from build123d import *

# Parameters (mm, degrees)
SKETCH1_W           = 160
SKETCH1_H           = 350
BOSS_EXTRUDE1_DEPTH = 3
SKETCH2_R           = 5
BOSS_EXTRUDE2_DEPTH = 20
SKETCH3_R           = 5
BOSS_EXTRUDE3_DEPTH = 20


with BuildPart() as part:
    # Sketch1 → Boss-Extrude1 (new body)
    with BuildSketch(Plane.XY):
        Rectangle(SKETCH1_W, SKETCH1_H)
    extrude(amount=BOSS_EXTRUDE1_DEPTH)

    # Sketch2 → Boss-Extrude2 (add)
    with BuildSketch(Plane.XY.offset(3)):
        with Locations((70, 150)):
            Circle(SKETCH2_R)
    boss_extrude2 = extrude(amount=BOSS_EXTRUDE2_DEPTH)

    # Mirror1: Boss-Extrude2 across plane
    add(boss_extrude2.mirror(Plane.ZX))

    # Sketch3 → Boss-Extrude3 (add)
    with BuildSketch(Plane.XY.offset(3)):
        with Locations((-60, 0)):
            Circle(SKETCH3_R)
    extrude(amount=BOSS_EXTRUDE3_DEPTH)


solid = part.part
Work out the finished part from the listing and answer in its coordinate system (mm). Round coordinates to 2 decimals unless told otherwise and drop trailing zeros. Write each loop counter-clockwise with the first axis right and the second up, starting at its lowest first coordinate (ties: lowest second). Pieces come first, ordered by that corner, then holes. Notation, with made-up numbers: (37.25, 40) -> (88.25, 40) arc R24 ccw to (88.25, 76) -> close; hole circle Ø7 at (12.25, 32.5). An arc over 180 degrees is marked (long way). Write each question's results on one line, items separated by ' | '.
Item 1: A cutting plane is placed at C-C, the plane x = 70. Determine the outline of the cut face in (y, z).
Result set:
outline: (-175, 0) -> (175, 0) -> (175, 3) -> (155, 3) -> (155, 23) -> (145, 23) -> (145, 3) -> (-145, 3) -> (-145, 23) -> (-155, 23) -> (-155, 3) -> (-175, 3) -> close
Item 2: A cutting plane is placed at B-B, the plane y = 150. Determine the outline of the cut face in (x, z), plus the area to 3 significant figures.
Result set:
outline: (-80, 0) -> (80, 0) -> (80, 3) -> (75, 3) -> (75, 23) -> (65, 23) -> (65, 3) -> (-80, 3) -> close | area: 680 mm^2
Item 3: A cutting plane is placed at D-D, the plane x = -60. Determine the outline of the cut face in (y, z), plus the area to 3 significant figures.
Result set:
outline: (-175, 0) -> (175, 0) -> (175, 3) -> (5, 3) -> (5, 23) -> (-5, 23) -> (-5, 3) -> (-175, 3) -> close | area: 1,250 mm^2
Item 4: The mould has two halves that part along Y. Classify faces 1 (the face through (-60, 0, 23)), 2 (the face through (74.619, 148.085, 12.86)), 3 (the face through (74.619, -148.085, 12.86)), 4 (the face through (-65, 0, 13)): +Y half, -Y half, draft (parallel to the pull), parting line (faces both ways), or undercut.
Result set:
face 1: draft | face 2: undercut | face 3: undercut | face 4: parting line
Item 5: Find the intervals of material crossed by line 1 along Z through (x, y) = (-13, 43.5); line 2 along Y through (x, z) = (67.5, 14.5); line 3 along Y through (x, z) = (-59, 17.25), in increasing order. Write a range as [from, to].
Result set:
line 1: [0, 3] | line 2: [-154.33, -145.67], [145.67, 154.33] | line 3: [-4.9, 4.9]
Item 6: A cutting plane is placed at A-A, the plane z = 16. Determine the outline of the cut face in (x, y).
Result set:
outline: circle Ø10 at (-60, 0); circle Ø10 at (70, -150); circle Ø10 at (70, 150)
Item 7: Flat-ended cylindrical pins translate along their axes: P1, Ø8, axis at y = 124, z = 4, coming from the -X side; P2, Ø6, axis at x = -14.5, z = 6.5, coming from the -Y side. Find the tip coordinate at first contact, or state that the pin passes through.
Result set:
P1: x = -80 | P2: through
